CAD build for the part. Positions are in the model's coordinates, mm. Face numbers are marked on the shaded views. A direction names the side the tool comes from. Round coordinates to 2 decimals unless told otherwise and drop trailing zeros. Order: outer loops, then holes, each group sorted by start corner. A loop starts at its lowest first (then second) coordinate and runs counter-clockwise, first axis right, second up. Notation, with made-up numbers: M 81.5,-13 L 140.5,-13 A11 ccw 140.5,1 Z; hole C 72,65 d5. An arc over 180 degrees is marked long. Answer as CSV lines item,"result". Start each with the question number.
Autodesk Inventor part; units mm, degrees
ref_plane "YZ Plane" through (0, 0, 0) normal (1, 0, 0) x (0, 1, 0)
ref_plane "XZ Plane" through (0, 0, 0) normal (0, 1, 0) x (-1, 0, 0)
ref_plane "XY Plane" through (0, 0, 0) normal (0, 0, 1) x (1, 0, 0)
sketch "Sketch1" plane through (0, 0, 0) normal (1, 0, 0) x (0, 1, 0)
  line L0 (0, 0) -> (0, 23.2432)
  line L1 (0, 23.2432) -> (0, 0)
  line L2 (0, 0) -> (17.5676, 0)
  line L3 (0, 0) -> (0, -18.1081)
  line L4 (0, 0) -> (-14.0541, 0)
  line L5 (-2.5, 10) -> (-2.5, -10)
  line L6 (-2.5, -10) -> (17.5, -10)
  line L7 (17.5, -10) -> (17.5, -5)
  line L8 (17.5, -5) -> (2.5, -5)
  line L9 (2.5, -5) -> (2.5, 10)
  line L10 (2.5, 10) -> (-2.5, 10)
  dimension "d0" = 20
  dimension "d1" = 5
  dimension "d2" = 5
  dimension "d3" = 20
extrude "Extrusion1" add sketch "Sketch1" along normal blind 15
sketch "Sketch2" plane through (0, -2.5, -10) normal (0, -1, 0) x (1, 0, 0)
  line L0 (0, 20) -> (0, 0)
  line L1 (0, 0) -> (15, 0)
  line L2 (15, 20) -> (15, 0)
  line L3 (0, 20) -> (15, 20)
  circle A0 centre (7.5, 12.5) radius 2.25
  point P0 (0, 10)
  dimension "d6" = 4.5
  dimension "d7" = 12.5
extrude "Extrusion2" cut sketch "Sketch2" against normal through all contours A0
sketch "Sketch3" plane through (0, 2.5, -5) normal (0, 0, 1) x (1, 0, 0)
  line L0 (0, 15) -> (0, 0)
  line L1 (0, 0) -> (15, 0)
  line L2 (15, 15) -> (15, 0)
  line L3 (0, 15) -> (15, 15)
  circle A0 centre (7.5, 7.5) radius 1.75
  point P0 (0, -2.5)
  dimension "d10" = 3.5
extrude "Extrusion3" cut sketch "Sketch3" against normal through all contours A0
chamfer "Chamfer1" distance 1.25 angle 45 1 edges at (5.75, 10, -5)
chamfer "Chamfer2" distance 1.5 angle 45 1 edges at (5.25, 2.5, 2.5)
fillet "Fillet1" radius 3 1 edges at (7.5, 2.5, -5)
fillet "Fillet2" radius 2 10 edges at (15, 0, 10) (15, 11.5, -5) (15, 2.5, 4) (15, 17.5, -7.5) (7.5, 2.5, 10) (0, 11.5, -5) (0, 2.5, 4) (7.5, 17.5, -5) (0, 0, 10) (0, 17.5, -7.5)
properties part number "escuadra"
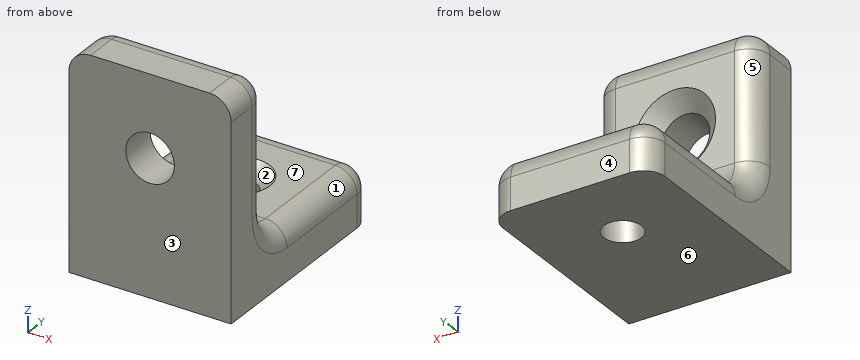
Q1. Band-saw the part on A-A, the plane z = 2.5. Write the cut outline in (x, y), then the cut area to 3 significant figures.
Q2. Band-saw the part on C-C, the plane x = 7.5. Write the cut outline in (y, z), then the cut area to 3 significant figures.
Q3. Drop flat-ended pins along their axis: P1, Ø5, axis at x = 7.5, z = 2.5, coming from the +Y side; P2, Ø3, axis at x = 5.5, y = 10.5, coming from the +Z side; P3, Ø3, axis at x = 7.5, y = 10, coming from the +Z side; P4, Ø4, axis at x = 7, z = 1, coming from the +Y side. Give the stop position or say it passes through.
Q4. Mould opens along Y. For the marked faces 1, 2, 3 and 4 say: +Y half, -Y half, draft (parallel to the pull), parting line (faces both ways), or undercut.
Q5. Band-saw the part on B-B, the plane y = 10. Write the cut outline in (x, z), then the cut area to 3 significant figures.
Q6. Tool access for the marked faces 5, 6 and 7: list every direction of +Z, -Z, +X, -X, +Y, -Y with a clear straight run to the whole face (end or side of a thin tool).
Q7. Band-saw the part on D-D, the plane x = 12.25. Write the cut outline in (y, z).
Q8. Probe line 1 along Y through (x, z) = (7.5, -8.8); line 2 along Z through (x, y) = (7.5, -0.5); line 3 along Y through (x, z) = (12, -1.75). List the from-to ranges inside material, lowest first. Write a range as from..to.
Answer:
1,outline,"M 0,-2.5 L 5.25,-2.5 L 5.25,1 L 3.75,2.5 L 2,2.5 A2 ccw 0,0.5 Z; M 9.75,-2.5 L 15,-2.5 L 15,0.5 A2 ccw 13,2.5 L 11.25,2.5 L 9.75,1 Z"
1,area,"48.5 mm^2"
2,outline,"M -2.5,-10 L 8.25,-10 L 8.25,-6.25 L 7,-5 L 5.5,-5 A3 cw 2.5,-2 L 2.5,-1.25 L 1,0.25 L -2.5,0.25 Z; M -2.5,4.75 L 1,4.75 L 2.5,6.25 L 2.5,8 A2 ccw 0.5,10 L -2.5,10 Z; M 11.75,-10 L 17.5,-10 L 17.5,-7 A2 ccw 15.5,-5 L 13,-5 L 11.75,-6.25 Z"
2,area,"131 mm^2"
3,P1,"stops at y = 1.25"
3,P2,"stops at z = -5"
3,P3,"passes through"
3,P4,"stops at y = 2.33"
4,face 1,"draft"
4,face 2,"undercut"
4,face 3,"-Y half"
4,face 4,"+Y half"
5,outline,"M 0,-10 L 5.75,-10 L 5.75,-6.25 L 4.5,-5 L 2,-5 A2 ccw 0,-7 Z; M 9.25,-10 L 15,-10 L 15,-7 A2 ccw 13,-5 L 10.5,-5 L 9.25,-6.25 Z"
5,area,"54.2 mm^2"
6,face 5,"+Z, -X, +Y"
6,face 6,"-Z, +X, -X, +Y, -Y"
6,face 7,"+Z, +X, -X, +Y"
7,outline,"M -2.5,-10 L 17.5,-10 L 17.5,-7 A2 ccw 15.5,-5 L 5.5,-5 A3 cw 2.5,-2 L 2.5,8 A2 ccw 0.5,10 L -2.5,10 Z"
8,line 1,"y = -2.5..8.25, 11.75..17.5"
8,line 2,"z = -10..0.25, 4.75..10"
8,line 3,"y = -2.5..2.5"
